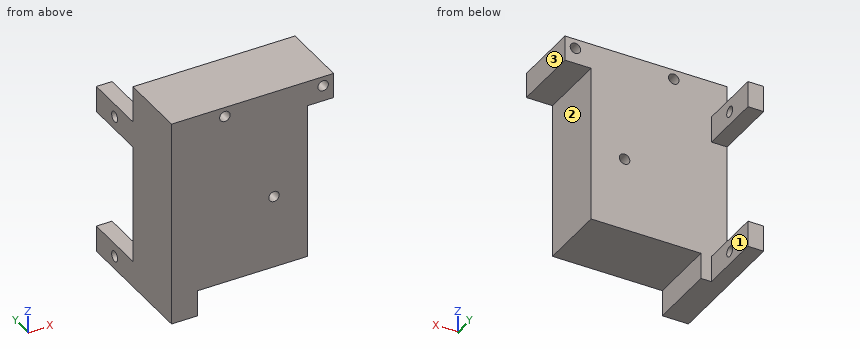
Autodesk Inventor part; units mm, degrees
ref_plane "YZ Plane" through (0, 0, 0) normal (1, 0, 0) x (0, 1, 0)
ref_plane "XZ Plane" through (0, 0, 0) normal (0, 1, 0) x (-1, 0, 0)
ref_plane "XY Plane" through (0, 0, 0) normal (0, 0, 1) x (1, 0, 0)
sketch "Sketch1" plane through (0, 0, 0) normal (0, 1, 0) x (-1, 0, 0)
  line L0 (9, -28.2161) -> (9, 11.5839)
  line L1 (9, 11.5839) -> (4, 11.5839)
  line L2 (4, 11.5839) -> (4, 11.5839)
  line L3 (4, 11.5839) -> (-22, 11.5839)
  line L4 (9, -28.2161) -> (4, -28.2161)
  line L5 (4, -28.2161) -> (4, -23.2161)
  line L6 (-22, 6.7839) -> (-22, 11.5839)
  line L7 (4, -23.2161) -> (-17, -23.2161)
  line L8 (-17, -23.2161) -> (-17, 6.7839)
  line L9 (-17, 6.7839) -> (-22, 6.7839)
  point P0 (0, 0)
  dimension "d28" = 0
  dimension "d30" = 5
  dimension "d69" = 5
  dimension "d98" = 5
  dimension "d101" = 21
  dimension "d102" = 30
extrude "Extrusion1" add sketch "Sketch1" along normal blind 13
sketch "Sketch7" plane through (0, 13, 0) normal (0, 1, 0) x (1, 0, 0)
  circle A0 centre (1.2, -9.7839) radius 1
  circle A1 centre (20, -9.7839) radius 1
  circle A2 centre (10.6, 9.2161) radius 1
  line L0 (22, 11.2161) -> (-4, 11.2161)
  line L1 (-9, 28.2161) -> (-9, -11.5839)
  line L2 (22, -11.5839) -> (22, 11.2161)
  point P0 (0, 0)
  point P1 (-4, 23.2161)
  point P2 (-9, 23.2161)
  point P3 (-9, -6.5839)
  dimension "d84" = 2
  dimension "d85" = 2
  dimension "d87" = 2
  dimension "d88" = 19
  dimension "d89" = 9.4
  dimension "d90" = 2
  dimension "d91" = 19
  dimension "d93" = 9.4
  dimension "d100" = 2
extrude "Extrusion8" cut sketch "Sketch7" against normal blind 15
sketch "Sketch8" plane through (0, 13, 0) normal (0, 1, 0) x (1, 0, 0)
  line L0 (-4, 28.2161) -> (-9, 28.2161)
  line L1 (-9, 28.2161) -> (-6, 28.2161)
  line L2 (-6, 28.2161) -> (-6, 23.2161)
  line L3 (-6, 23.2161) -> (-9, 23.2161)
  line L4 (-9, 23.2161) -> (-9, 28.2161)
  line L5 (-9, 28.2161) -> (-9, -11.5839)
  line L6 (-6, -4.5839) -> (-9, -4.5839)
  line L7 (-9, -4.5839) -> (-9, 0.4161)
  line L8 (-9, 0.4161) -> (-6, 0.4161)
  line L9 (-6, 0.4161) -> (-6, -4.5839)
  point P0 (0, 0)
  dimension "d103" = 3
  dimension "d104" = 5
  dimension "d105" = 5
  dimension "d106" = 3
  dimension "d107" = 22.8
extrude "Extrusion9" add sketch "Sketch8" along normal blind 12.3
sketch "Sketch9" plane through (-9, 0, -28.2161) normal (-1, 0, 0) x (0, 0, 1)
  circle A0 centre (30.3, 19.15) radius 1
  line L0 (32.8, 13) -> (32.8, 25.3)
  line L1 (32.8, 13) -> (39.8, 13)
  circle A1 centre (2.5, 19.15) radius 1
  line L2 (5, 13) -> (27.8, 13)
  line L3 (5, 13) -> (5, 25.3)
  point P0 (28.2161, 0)
  dimension "d110" = 2
  dimension "d111" = 2.5
  dimension "d112" = 6.15
  dimension "d113" = 2
  dimension "d114" = 6.15
  dimension "d115" = 2.5
extrude "Extrusion10" cut sketch "Sketch9" against normal blind 12.3
properties part number "spojene 2"
Can you work these out from the model? Positions are in its coordinate system, mm. Face numbers are marked on the shaded views. A direction names the side the tool comes from. Give positions to 0.01 mm unless a question says otherwise; leave off trailing zeros. Loops run counter-clockwise (first coordinate to the right, second up) from the corner with the lowest first, then second, coordinate; pieces in that order, holes last. Notation, with made-up numbers: M 72.5,61.5 L 76.5,61.5 A27 ccw 76.5,93.5 Z; hole C 57,64.25 d9. An arc over 180 degrees is marked long. One line per question, with ' | ' between items. Start each with the question number.
Q1. If we section it at C-C (y = 3.5): Please give me the cut outline in (x, z), plus the area to 3 significant figures.
Q2. For the marked faces 1, 2 and 3, which set-ups out of +Z, -Z, +X, -X, +Y, -Y let a thin tool reach every point of the face, with its end or its side?
Q3. If I drill on line 1 (Z direction, x = -7.5, y = 13.25); line 2 (Z direction, x = 20, y = 8.5); line 3 (X direction, y = 9.5, z = 2.5), over which ranges is the centre line in solid material (lowest first)? Write a range as from..to.
Q4. If we section it at A-A (y = 19.15): Please give me the cut outline in (x, z), plus the area to 3 significant figures.
Q5. If we section it at B-B (x = 20): Please give me the cut outline in (y, z).
Q6. For pin 1 Ø8 at (x, y) = (4, 10.5) entering from -Z; pin 2 Ø6.5 at (y, z) = (8.5, -2.5) entering from +X; pin 3 Ø4 at (y, z) = (22, 2) entering from +X; pin 4 Ø1.8 at (y, z) = (19.15, 2.08) entering from -X, each with a flat end and sliding along its axis, tell me the tip position at first contact or that it passes through.
Q7. If we section it at D-D (z = -24): Please give me the cut outline in (x, y).
Computed:
1) outline: M -9,-28.22 L -4,-28.22 L -4,-23.22 L 17,-23.22 L 17,6.78 L 22,6.78 L 22,11.58 L -9,11.58 Z; hole C 1.2,9.78 d2; hole C 10.6,-9.22 d2; hole C 20,9.78 d2 | area: 944 mm²
2) face 1: +Z, -Z, +X, +Y | face 2: -Z, +X, +Y, -Y | face 3: +Z, -Z, +X, +Y, -Y
3) line 1: z = -28.22..-23.22, -0.42..4.58 | line 2: z = 6.78..8.78, 10.78..11.58 | line 3: x = -9..17
4) outline: M -9,-28.22 L -6,-28.22 L -6,-26.72 L -9,-26.72 Z; M -9,-24.72 L -6,-24.72 L -6,-23.22 L -9,-23.22 Z; M -9,-0.42 L -6,-0.42 L -6,1.08 L -9,1.08 Z; M -9,3.08 L -6,3.08 L -6,4.58 L -9,4.58 Z | area: 18.0 mm²
5) outline: M 0,6.78 L 13,6.78 L 13,8.78 L 0,8.78 Z; M 0,10.78 L 13,10.78 L 13,11.58 L 0,11.58 Z
6) pin 1: stops at z = -23.22 | pin 2: stops at x = 17 | pin 3: stops at x = -6 | pin 4: passes through
7) outline: M -9,0 L -4,0 L -4,13 L -6,13 L -6,25.3 L -9,25.3 Z
